Geometry: final body of the model. Coordinates: model frame, mm. Give positions to 0.01 mm unless a question says otherwise; leave off trailing zeros. Order: outer loops, then holes, each group sorted by start corner. A loop starts at its lowest first (then second) coordinate and runs counter-clockwise, first axis right, second up. Notation, with made-up numbers: (5.5, -11.5) -> (34.5, -11.5) arc R21 ccw to (34.5, 2.5) -> close; hole circle Ø1 at (-2.5, 23.25). An arc over 180 degrees is marked (long way). One line per question, with ' | ' between items.
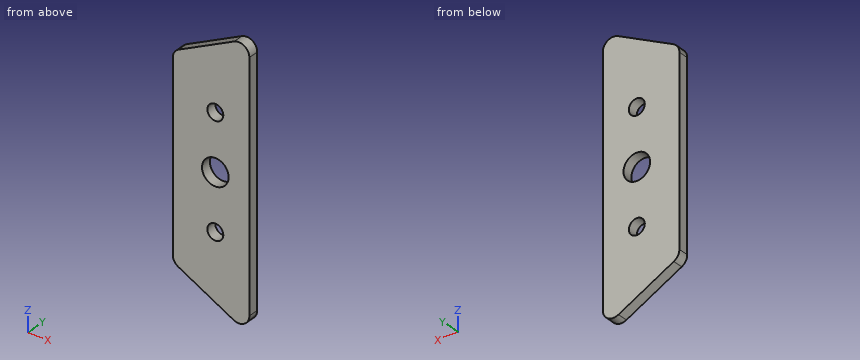
Autodesk Inventor part; units mm, degrees
ref_plane "YZ Plane" through (0, 0, 0) normal (1, 0, 0) x (0, 1, 0)
ref_plane "XZ Plane" through (0, 0, 0) normal (0, 1, 0) x (-1, 0, 0)
ref_plane "XY Plane" through (0, 0, 0) normal (0, 0, 1) x (1, 0, 0)
sketch "Sketch1" plane through (0, 0, 0) normal (0, 1, 0) x (-1, 0, 0)
  circle A0 centre (0, 0) radius 3.9688
  circle A1 centre (0, -16.6624) radius 2.3813
  circle A2 centre (0, 16.6624) radius 2.3813
  line L0 (12.7, 27.4344) -> (12.7, -27.4344)
  line L1 (-10.16, 35.4975) -> (-10.16, -36.4279)
  line L2 (10.9183, 30.2873) -> (-5.5917, 38.3505)
  line L3 (12.7, 29.4172) -> (45.9346, 29.4172) construction
  line L4 (-10.16, -0.5957) -> (-17.3723, -0.5957) construction
  line L5 (11.0438, -30.2225) -> (-5.4662, -39.2161)
  arc A3 (-5.5917, 38.3505) -> (-10.16, 35.4975) centre (-6.985, 35.4975) ccw
  arc A4 (12.7, 27.4344) -> (10.9183, 30.2873) centre (9.525, 27.4344) ccw
  arc A5 (11.0438, -30.2225) -> (12.7, -27.4344) centre (9.525, -27.4344) ccw
  arc A6 (-10.16, -36.4279) -> (-5.4662, -39.2161) centre (-6.985, -36.4279) ccw
  point P0 (12.7, -29.3203)
  point P1 (12.7, 0)
  point P2 (-10.16, -41.773)
  point P3 (-10.16, 40.5816)
  dimension "d0" = 7.9375
  dimension "d1" = 4.7625
  dimension "d2" = 16.6624
  dimension "d3" = 4.7625
  dimension "d4" = 16.6624
  dimension "d5" = 12.7
  dimension "d6" = 58.7375
  dimension "d7" = 22.86
  dimension "d8" = 153.97
  dimension "d9" = 3.175
extrude "Extrusion1" add sketch "Sketch1" along normal blind 3.175
properties part number "Bumper_Lock_Plate"
1) Section C-C on x = 0. Return loops of the section in (y, z) (3 decimals), plus the area to 3 significant figures.
Check result:
outline: (0, -36.238) -> (3.175, -36.238) -> (3.175, -19.044) -> (0, -19.044) -> close; (0, -14.281) -> (3.175, -14.281) -> (3.175, -3.969) -> (0, -3.969) -> close; (0, 3.969) -> (3.175, 3.969) -> (3.175, 14.281) -> (0, 14.281) -> close; (0, 19.044) -> (3.175, 19.044) -> (3.175, 35.62) -> (0, 35.62) -> close | area: 173 mm^2
2) Material intervals for probe 1 along Z at (x, y) = (0, 1.5); probe 2 along Z at (x, y) = (-2, 0.7); probe 3 along X at (y, z) = (0.5, 17.5), sorted ascending. Write a range as from..to.
Check result:
probe 1: z = -36.24..-19.04, -14.28..-3.97, 3.97..14.28, 19.04..35.62 | probe 2: z = -35.15..-17.95, -15.37..-3.43, 3.43..15.37, 17.95..34.64 | probe 3: x = -12.7..-2.23, 2.23..10.16
3) Section D-D on z = -18. Return loops of the section in (x, y) (3 decimals).
Check result:
outline: (-12.7, 0) -> (-1.97, 0) -> (-1.97, 3.175) -> (-12.7, 3.175) -> close; (1.97, 0) -> (10.16, 0) -> (10.16, 3.175) -> (1.97, 3.175) -> close
4) Section B-B on y = 1.1. Count the separate pieces of the cut face and the enclosed holes in it, plus the area to 3 significant figures.
Check result:
separate pieces: 1 | enclosed holes: 3 | area: 1,510 mm^2
5) Section A-A on z = 0. Return loops of the section in (x, y) (3 decimals), plus the area to 3 significant figures.
Check result:
outline: (-12.7, 0) -> (-3.969, 0) -> (-3.969, 3.175) -> (-12.7, 3.175) -> close; (3.969, 0) -> (10.16, 0) -> (10.16, 3.175) -> (3.969, 3.175) -> close | area: 47.4 mm^2
